Study the drawing (mm; zero at the part's minimum x, y, z) and answer. A direction names the side the tool comes from. Round coordinates to 2 decimals unless told otherwise and drop trailing zeros. Write each loop counter-clockwise with the first axis right and the second up, starting at its lowest first coordinate (ties: lowest second). Pieces come first, ordered by that corner, then holes. Notation, with made-up numbers: (-0.75, 77) - (43.25, 77) arc R26 cw to (43.25, 116) - close; hole circle Ø7 at (88.25, -7). An arc over 180 degrees is marked (long way). Return JSON: item names as keys, results as strings. Group by question number.
(1) Section C-C, the plane z = 10.5 is taken. Write down the section's boundary in (x, y), then the cut area to 3 significant figures.
(2) Determine the mould class of the marked faces 1 and 2 for opening direction Y: +Y half, -Y half, draft (parallel to the pull), parting line (faces both ways), or undercut.
(3) Find the intervals of material crossed by line 1 along Z through (x, y) = (41, 44); line 2 along Z through (x, y) = (55, 26); line 3 along Y through (x, z) = (53.5, 29.5), in increasing order. Write a range as [from, to].
(4) Each of these flat-tipped pins is pushed along its axis until it touches: pin 1 (1.5 mm diameter, centred on x = 21.5, z = 23, fed in from -Y); pin 2 (1 mm diameter, centred on x = 35.5, z = 34.5, fed in from -Y); pin 3 (6 mm diameter, centred on x = 7, z = 60, fed in from -Y). Where does it stop, or does it pass through?
(5) Section D-D, the plane z = 72 is taken. Write down the section's boundary in (x, y).
(6) Which of the six approach directions +Z, -Z, +X, -X, +Y, -Y give full straight-line access (tool end or side, diameter ignored) to the marked faces 3 and 4?
(7) Section A-A, the plane y = 30 is taken. Write down the section's boundary in (x, z).
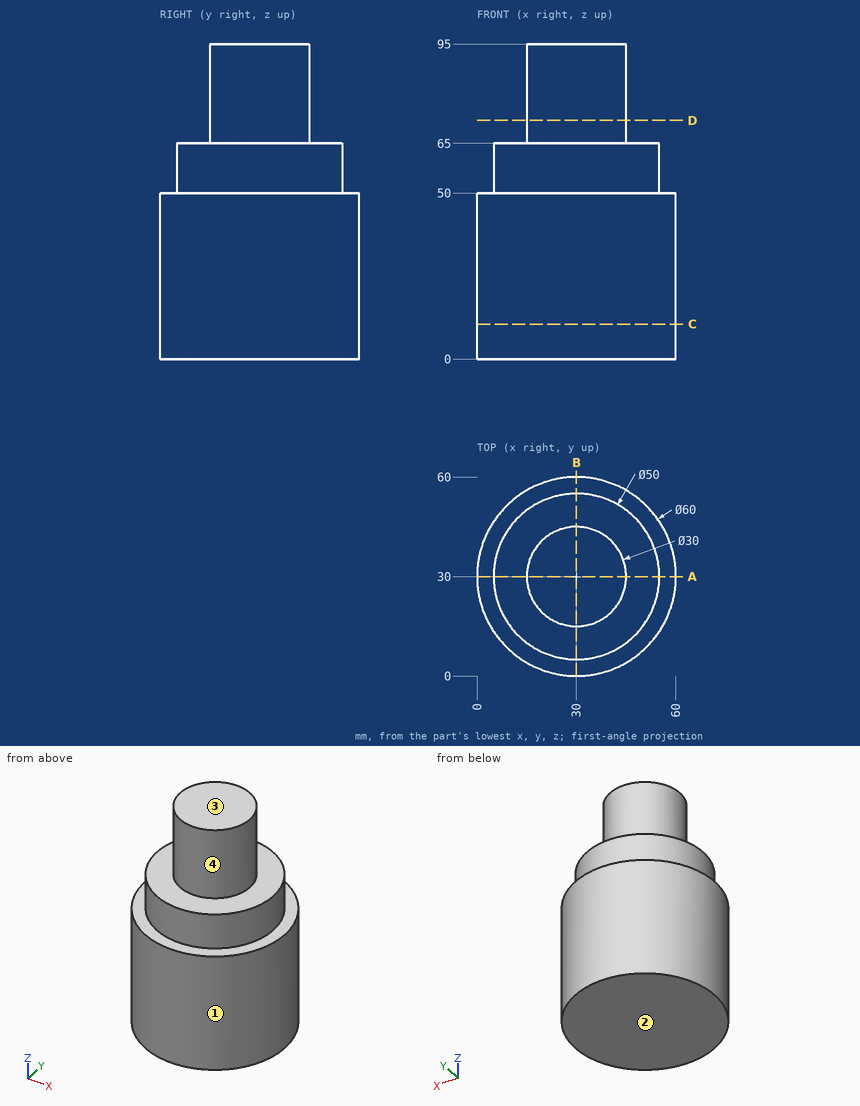
Working result:
{
 "1": {"outline": "circle Ø60 at (30, 30)", "area": "2,830 mm^2"},
 "2": {"face 1": "parting line", "face 2": "draft"},
 "3": {"line 1": "z = [0, 65]", "line 2": "z = [0, 50]", "line 3": "y = [11.35, 48.65]"},
 "4": {"pin 1": "stops at y = 1.02", "pin 2": "stops at y = 0.42", "pin 3": "stops at y = 15"},
 "5": {"outline": "circle Ø30 at (30, 30)"},
 "6": {"face 3": "+Z, +X, -X, +Y, -Y", "face 4": "+Z"},
 "7": {"outline": "(0, 0) - (60, 0) - (60, 50) - (55, 50) - (55, 65) - (45, 65) - (45, 95) - (15, 95) - (15, 65) - (5, 65) - (5, 50) - (0, 50) - close"}
}
